Autodesk Inventor part; units mm, degrees
ref_plane "YZ Plane" through (0, 0, 0) normal (1, 0, 0) x (0, 1, 0)
ref_plane "XZ Plane" through (0, 0, 0) normal (0, 1, 0) x (-1, 0, 0)
ref_plane "XY Plane" through (0, 0, 0) normal (0, 0, 1) x (1, 0, 0)
sketch "Эскиз1" plane through (0, 0, 0) normal (1, 0, 0) x (0, 1, 0)
  line L0 (-4, 19) -> (4, 19)
  line L1 (4, 19) -> (4, -19)
  line L2 (4, -19) -> (-4, -19)
  line L3 (-4, -19) -> (-4, 19)
  line L4 (-4, 19) -> (4, -19) construction
  line L5 (4, 19) -> (-4, -19) construction
  point P0 (0, 0)
  dimension "d0" = 8
  dimension "d1" = 38
extrude "Выдавливание1" add sketch "Эскиз1" along normal blind 20.2
sketch "Эскиз2" plane through (0, 0, 0) normal (-1, 0, 0) x (0, 0, 1)
  line L0 (0, 0) -> (-15, 0)
  line L1 (0, 0) -> (15, 0) construction
  line L2 (-15, 0) -> (15, 0)
  circle A0 centre (-15, 0) radius 1.5
  circle A1 centre (15, 0) radius 1.5
  dimension "d4" = 15
  dimension "d5" = 180
  dimension "d6" = 30
  dimension "d7" = 3
  dimension "d8" = 3
extrude "Выдавливание2" cut sketch "Эскиз2" against normal through all
sketch "Эскиз3" plane through (0, -4, -19) normal (0, -1, 0) x (1, 0, 0)
  line L0 (0, 38) -> (20.2, 38)
  line L1 (0, 0) -> (20.2, 0)
  line L2 (20.2, 38) -> (12.4, 38)
  line L3 (12.4, 38) -> (12.4, 0)
  line L4 (12.4, 0) -> (20.2, 0)
  line L5 (20.2, 0) -> (20.2, 38)
  point P0 (0, 19)
  dimension "d11" = 7.8
extrude "Выдавливание3" add sketch "Эскиз3" along normal blind 8
sketch "Эскиз4" plane through (20.2, 0, 0) normal (1, 0, 0) x (0, 0, -1)
  line L0 (19, -4) -> (-19, -4)
  line L1 (-18.1844, -4) -> (0, -4)
  line L2 (19, 4) -> (-19, 4)
  line L3 (-11, -4) -> (11, -4)
  line L4 (11, -4) -> (11, 4)
  line L5 (11, 4) -> (-11, 4)
  line L6 (-11, 4) -> (-11, -4)
  line L7 (-11, -4) -> (11, 4) construction
  line L8 (11, -4) -> (-11, 4) construction
  point P0 (0, 0)
  dimension "d17" = 22
extrude "Выдавливание4" add sketch "Эскиз4" along normal blind 9.8
sketch "Эскиз5" plane through (0, 4, 19) normal (0, 1, 0) x (1, 0, 0)
  line L0 (0, 38) -> (12.4, 38)
  line L1 (12.4, 38) -> (24.4, 38)
  line L2 (24.4, 38) -> (24.4, 0)
  line L3 (24.4, 0) -> (12.4, 0)
  line L4 (12.4, 0) -> (12.4, 38)
  line L5 (20.2, 8) -> (30, 8)
  line L6 (20.2, 38) -> (20.2, 0)
  line L7 (24.4, 8) -> (20.2, 8)
  line L8 (20.2, 8) -> (20.2, 30)
  line L9 (20.2, 30) -> (24.4, 30)
  line L10 (24.4, 30) -> (24.4, 8)
  line L11 (12.4, 0) -> (12.4, 38)
  line L12 (12.4, 8) -> (8.2, 8)
  line L13 (8.2, 8) -> (8.2, 30)
  line L14 (8.2, 30) -> (12.4, 30)
  line L15 (12.4, 30) -> (12.4, 8)
  point P0 (0, 19)
  dimension "d20" = 12
  dimension "d21" = 38
  dimension "d24" = 22
  dimension "d25" = 4.2
  dimension "d26" = 4.2
extrude "Выдавливание5" cut sketch "Эскиз5" against normal blind 1
sketch "Эскиз6" plane through (0, 3, 19) normal (0, 1, 0) x (1, 0, 0)
  circle A0 centre (10.1672, 27.1433) radius 1.5
  circle A1 centre (10.1672, 10.008) radius 1.5
  circle A2 centre (22.0732, 27.1433) radius 1.5
  circle A3 centre (22.0732, 10.008) radius 1.5
  point P0 (0, 19)
  dimension "d27" = 3
  dimension "d28" = 3
  dimension "d29" = 3
  dimension "d30" = 3
extrude "Выдавливание6" cut sketch "Эскиз6" against normal blind 4.5
sketch "Эскиз7" plane through (0, 3, 19) normal (0, 1, 0) x (1, 0, 0)
  circle A0 centre (22.0732, 27.1433) radius 1.5
  circle A1 centre (10.1672, 27.1433) radius 1.5
  circle A2 centre (10.1672, 10.008) radius 1.5
  circle A3 centre (22.0732, 10.008) radius 1.5
  line L0 (20.2, 8) -> (20.2, 0)
  line L1 (24.4, 8) -> (20.2, 8)
  line L2 (24.4, 30) -> (24.4, 8)
  line L3 (20.2, 30) -> (24.4, 30)
  line L4 (20.2, 38) -> (20.2, 30)
  line L5 (12.4, 38) -> (20.2, 38)
  line L6 (12.4, 30) -> (12.4, 38)
  line L7 (8.2, 30) -> (12.4, 30)
  line L8 (8.2, 8) -> (8.2, 30)
  line L9 (12.4, 8) -> (8.2, 8)
  line L10 (12.4, 0) -> (12.4, 8)
  line L11 (20.2, 0) -> (12.4, 0)
  point P0 (0, 19)
properties part number "КВ33.044.502 - Фиксатор оси Y" material "Пластик АБС"
Work out the finished part from the listing and answer in its coordinate system (mm). A direction names the side the tool comes from. Round coordinates to 2 decimals unless told otherwise and drop trailing zeros. Loops run counter-clockwise (first coordinate to the right, second up) from the corner with the lowest first, then second, coordinate; pieces in that order, holes last.
(1) For faces 4 (the flat face through (10, -1.5, 9)), 5 (the flat face through (12.4, 3.5, 15.1)), 6 (the flat face through (16, -12, 0)), 7 (the flat face through (12.4, -8, 0)), 8 (the cylindrical face through (9.96, 0.07, 13.5)), determine the directions among +Z, -Z, +X, -X, +Y, -Y from which every point of the face is accessible in a straight line to the end or side of a thin tool.
Computed values:
face 4: +Y
face 5: +Z, -Z, +X, +Y
face 6: +Z, -Z, +X, -X, -Y
face 7: +Z, -Z, -X, -Y
face 8: +X, -X
(2) The part is cut by section B-B, the plane z = -15. Give the vertices of the cut face in (x, y).
Computed values:
outline: (0, -4) - (12.4, -4) - (12.4, -12) - (20.2, -12) - (20.2, -1.5) - (0, -1.5) - close; (0, 1.5) - (20.2, 1.5) - (20.2, 3) - (12.4, 3) - (12.4, 4) - (0, 4) - close
(3) The part is cut by section D-D, the plane x = 14.5. Give the vertices of the cut face in (y, z).
Computed values:
outline: (-12, -19) - (3, -19) - (3, 19) - (-12, 19) - close; hole circle Ø3 at (0, -15); hole circle Ø3 at (0, 15)
(4) Each of these flat-tipped pins is pushed along its axis until it touches: P1, Ø4, axis at y = -4, z = 8, coming from the -X side; P2, Ø2.5, axis at x = 10.17, z = 8.99, coming from the -Y side; P3, Ø1, axis at y = 1, z = 12.5, coming from the +X side; P4, Ø4, axis at y = -7.5, z = -7, coming from the -X side. Where does it stop, or does it pass through?
Computed values:
P1: stops at x = 0
P2: stops at y = -4
P3: stops at x = 20.2
P4: stops at x = 12.4
(5) Find the intervals of material crossed by L1, parallel to Y at x = 14.75, z = -15; L2, parallel to X at y = -0.25, z = 10; L3, parallel to Y at x = 5, z = 15, in increasing order.
Computed values:
L1: y = -12 to -1.5, 1.5 to 3
L2: x = 0 to 9.06, 11.28 to 20.96, 23.18 to 30
L3: y = -4 to -1.5, 1.5 to 4
(6) The mould has two halves that part along X. Classify faces 1 (the flat face through (22, -1.5, -8)), 2 (the flat face through (30, 0, 0)), 3 (the flat face through (25, 0, 11)): pulls with the +X half, pulls with the -X half, needs draft (parallel to the pull), parting line crosses it, or undercut.
Computed values:
face 1: undercut
face 2: pulls with the +X half
face 3: needs draft
(7) The part is cut by section A-A, the plane y = 0. Give the vertices of the cut face in (x, z), and give its area (3 significant figures).
Computed values:
outline: (0, -19) - (20.2, -19) - (20.2, -16.5) - (0, -16.5) - close; (0, -13.5) - (20.2, -13.5) - (20.2, -11) - (30, -11) - (30, 11) - (20.2, 11) - (20.2, 13.5) - (0, 13.5) - close; (0, 16.5) - (20.2, 16.5) - (20.2, 19) - (0, 19) - close; hole circle Ø3 at (10.17, -8.14); hole circle Ø3 at (10.17, 8.99); hole circle Ø3 at (22.07, -8.14); hole circle Ø3 at (22.07, 8.99)
area: 834 mm2
(8) The part is cut by section C-C, the plane z = -0.5. Give the vertices of the cut face in (x, y).
Computed values:
outline: (0, -4) - (12.4, -4) - (12.4, -12) - (20.2, -12) - (20.2, -4) - (30, -4) - (30, 4) - (24.4, 4) - (24.4, 3) - (8.2, 3) - (8.2, 4) - (0, 4) - close
